For this review, take the finished solid that the model builds, in its own axes (mm). A direction names the side the tool comes from. Coordinates: 2 decimals unless noted, no trailing zeros. Order: outer loops, then holes, each group sorted by start corner. A loop starts at its lowest first (then second) coordinate and runs counter-clockwise, first axis right, second up. Notation, with made-up numbers: (17.5, -7.75) -> (73.5, -7.75) arc R23 cw to (73.5, 23.25) -> close; hole circle Ø10 at (16, 5). An arc over 180 degrees is marked (long way). Return JSON: item names as keys, results as strings. Group by question number.
Item 1: Take a section at D-D (z = 12). Write out the cut boundary in (x, y).
Item 2: Take a section at C-C (x = -34). Write out the cut boundary in (y, z), then the cut area to 3 significant figures.
Item 3: Insertion check: pin 1 (12 mm diameter, centred on x = -22, z = -1.5, fed in from +Y); pin 2 (22 mm diameter, centred on y = -14, z = 3, fed in from -X); pin 3 (10 mm diameter, centred on x = -20.5, y = 18, fed in from -Z); pin 4 (3 mm diameter, centred on y = 3.5, z = -4, fed in from -X). Each pin has a flat end and moves straight along its axis. Give the tip position at first contact, or say it passes through.
Item 4: Draft analysis for pull direction Z (two halves, no side actions). For faces 1 (the cylindrical face through (-49.76, 22.4, -2.17)), 2 (the flat face through (-9, 15, 0)), 3 (the cylindrical face through (-35.043, 14.79, -0.651)), 4 (the flat face through (-1, 6, 20)), state which applies: +Z half, -Z half, draft (parallel to the pull), parting line (faces both ways), or undercut.
Item 5: For line 1 along X through (y, z) = (16, 0); line 2 along Y through (x, z) = (-22.5, -9); line 3 along X through (y, z) = (-12, 4.5), list the stretches that pass through material, from the lowest coordinate up.
Item 6: Take a section at A-A (z = 0). Write out the cut boundary in (x, y), then the cut area to 3 significant figures.
Item 7: Take a section at B-B (y = 12.5). Write out the cut boundary in (x, z).
Item 8: Machinability: for faces 5 (the flat face through (-14, 0, 0)), 6 (the flat face through (40, -2, 0)), which of the approach directions +Z, -Z, +X, -X, +Y, -Y give a long, thin tool a straight path to every point of the face, cutting with its end or side? Answer none if there is none.
```python
from build123d import *

# Parameters (mm, degrees)
CROQUIS2_R              = 5
SALIENTE_EXTRUIR1_DEPTH = 15
CROQUIS3_R              = 10
CROQUIS3_R_2            = 5
SALIENTE_EXTRUIR2_DEPTH = 15
CROQUIS4_W              = 10
CROQUIS4_H              = 40
SALIENTE_EXTRUIR3_DEPTH = 20


with BuildPart() as part:
    # Croquis2 → Saliente-Extruir1 (new body)
    with BuildSketch(Plane(origin=(0, 0, 0), x_dir=(1, 0, 0), z_dir=(0, 1, 0))):
        with BuildLine():
            Line((-40, 20), (40, 20))
            Line((40, 20), (40, -20))
            Line((40, -20), (-40, -20))
            ThreePointArc((-40, -20), (-60, 0), (-40, 20))
        make_face()
        with Locations(Location((-40, 0, 0), (0, 0, 270))):
            Circle(CROQUIS2_R, mode=Mode.SUBTRACT)
    extrude(amount=SALIENTE_EXTRUIR1_DEPTH)

    # Croquis3 → Saliente-Extruir2 (add)
    with BuildSketch(Plane(origin=(0, 15, 0), x_dir=(1, 0, 0), z_dir=(0, 1, 0))):
        with Locations(Location((-40, 0, 0), (0, 0, 270))):
            Circle(CROQUIS3_R)
        with Locations(Location((-40, 0, 0), (0, 0, 270))):
            Circle(CROQUIS3_R_2, mode=Mode.SUBTRACT)
    extrude(amount=SALIENTE_EXTRUIR2_DEPTH)

    # Croquis4 → Saliente-Extruir3 (add)
    with BuildSketch(Plane.XZ):
        with Locations((35, 0)):
            Rectangle(CROQUIS4_W, CROQUIS4_H)
    extrude(amount=SALIENTE_EXTRUIR3_DEPTH)


solid = part.part
```
Findings below:
{
 "1": {"outline": "(-56, 0) -> (30, 0) -> (30, -20) -> (40, -20) -> (40, 15) -> (-56, 15) -> close"},
 "2": {"outline": "(0, -20) -> (15, -20) -> (15, -8) -> (30, -8) -> (30, 8) -> (15, 8) -> (15, 20) -> (0, 20) -> close", "area": "840 mm2"},
 "3": {"pin 1": "stops at y = 15", "pin 2": "stops at x = 30", "pin 3": "stops at z = -20", "pin 4": "stops at x = -59.84"},
 "4": {"face 1": "parting line", "face 2": "draft", "face 3": "undercut", "face 4": "+Z half"},
 "5": {"line 1": "x = -50 to -45, -35 to -30", "line 2": "y = 0 to 15", "line 3": "x = 30 to 40"},
 "6": {"outline": "(-60, 0) -> (-45, 0) -> (-45, 30) -> (-50, 30) -> (-50, 15) -> (-60, 15) -> close; (-35, 0) -> (30, 0) -> (30, -20) -> (40, -20) -> (40, 15) -> (-30, 15) -> (-30, 30) -> (-35, 30) -> close", "area": "1,700 mm2"},
 "7": {"outline": "(-40, -20) -> (40, -20) -> (40, 20) -> (-40, 20) arc R20 ccw to start; hole circle Ø10 at (-40, 0)"},
 "8": {"face 5": "+Z, -Z, -X, -Y", "face 6": "+Z, -Z, +X, +Y, -Y"}
}
